Verification items for the finished model (mm, model axes). Coordinates: 2 decimals unless noted, no trailing zeros. Write each loop counter-clockwise with the first axis right and the second up, starting at its lowest first coordinate (ties: lowest second). Pieces come first, ordered by that corner, then holes. Notation, with made-up numbers: (-4.5, -10) -> (18.5, -10) arc R27 cw to (18.5, 14) -> close; hole circle Ø3 at (5, 71). An arc over 180 degrees is marked (long way). Write each question's results on one line, items separated by ' | '. Start each with the question number.
from build123d import *

# Parameters (mm, degrees)
F0_W     = 29
F0_H     = 29
F0_R     = 10.5
F0_R_2   = 7.5
F3_DEPTH = 24
F2_R     = 10.5
F5_DEPTH = 1
F6_DEPTH = 2


with BuildPart() as f3:
    # F0 (on Top) → F3 (new body, through all)
    with BuildSketch(Plane.XY):
        Rectangle(F0_W, F0_H)
        Circle(F0_R, mode=Mode.SUBTRACT)
        Circle(F0_R)
        Circle(F0_R_2, mode=Mode.SUBTRACT)
    extrude(amount=F3_DEPTH)

    # F0 (on Top) → F4 section 0
    with BuildSketch(Plane.XY):
        Circle(F0_R_2)
    # F2 (on offset) → F4 section 1
    with BuildSketch(Plane.XY.offset(24)):
        Circle(F2_R)
    loft(mode=Mode.SUBTRACT)

    # F0 (on Top) → F5 (join)
    with BuildSketch(Plane.XY):
        Rectangle(F0_W, F0_H)
        Circle(F0_R, mode=Mode.SUBTRACT)
        Circle(F0_R)
        Circle(F0_R_2, mode=Mode.SUBTRACT)
    extrude(amount=-F5_DEPTH)

    # F0 (on Top) → F6 (join)
    with BuildSketch(Plane.XY):
        Rectangle(F0_W, F0_H)
        Circle(F0_R, mode=Mode.SUBTRACT)
        Circle(F0_R)
        Circle(F0_R_2, mode=Mode.SUBTRACT)
        Circle(F0_R_2)
    extrude(amount=-F6_DEPTH)


solid = f3.part
1. Sectioned sample at A-A on x = 0. Record the cut outline in (y, z), plus the area to 3 significant figures.
2. Sectioned sample at B-B on z = 12. Record the cut outline in (x, y).
3. Sectioned sample at C-C on z = 4. Record the cut outline in (x, y).
4. Mould release check, pull along Y, two halves, no side actions. Record for faces 1 (the conical face through (-9, 0, 12)), 2 (the flat face through (0, -14.5, 11)), 3 (the flat face through (-14.5, 0, 11)), 4 (the flat face through (0, 0, 0)): +Y half, -Y half, draft (parallel to the pull), parting line (faces both ways), or undercut.
5. Material ranges on probe 1 along Z at (x, y) = (4.75, 5.25); probe 2 along X at (y, z) = (3.75, 16.25); probe 3 along Y at (x, z) = (-7.25, 17), recorded low to high. Write a range as from..to.
6. Depth check by flat-ended pin: pin 1 Ø7.5 at (x, y) = (-2, -1) entering from +Z. Enter the tip coordinate at first touch or a pass-through.
Computed values:
1) outline: (-14.5, -2) -> (14.5, -2) -> (14.5, 24) -> (10.5, 24) -> (7.5, 0) -> (-7.5, 0) -> (-10.5, 24) -> (-14.5, 24) -> close | area: 322 mm^2
2) outline: (-14.5, -14.5) -> (14.5, -14.5) -> (14.5, 14.5) -> (-14.5, 14.5) -> close; hole circle Ø18 at (0, 0)
3) outline: (-14.5, -14.5) -> (14.5, -14.5) -> (14.5, 14.5) -> (-14.5, 14.5) -> close; hole circle Ø16 at (0, 0)
4) face 1: undercut | face 2: -Y half | face 3: draft | face 4: undercut
5) probe 1: z = -2..0 | probe 2: x = -14.5..-8.76, 8.76..14.5 | probe 3: y = -14.5..-6.33, 6.33..14.5
6) pin 1: stops at z = 0
